Check sheet for the modelled part. Datum: model origin and axes. Units: mm. A direction names the side the tool comes from. Give positions to 0.01 mm unless a question says otherwise; leave off trailing zeros. Loops run counter-clockwise (first coordinate to the right, second up) from the corner with the lowest first, then second, coordinate; pieces in that order, holes last. Notation, with made-up numbers: (31, -18) -> (35, -18) arc R21 cw to (35, -1) -> close; hole circle Ø11 at (41, 33.5). An arc over 180 degrees is marked (long way). Write each question's results on one line, items separated by ' | '. Start each with the question number.
Item 1: Scan lines: line 1 along Z through (x, y) = (-4, 5); line 2 along Z through (x, y) = (12.5, 32.5); line 3 along X through (y, z) = (3.5, 3.75). Record each from-to range of solid material in increasing order.
Item 2: Cross-section at B-B on y = 37.5. Enter the section's corners in (x, z).
Item 3: Cross-section at A-A on x = 14. Enter the section's corners in (y, z).
Item 4: Cross-section at D-D on x = -2. Enter the section's corners in (y, z).
Item 5: Access from +Z, -Z, +X, -X, +Y, -Y to the whole of each face (thin tool, end or side, straight path). Record for faces 1 (the face through (0, 31, -8.25)), 2 (the face through (14, 22, -14.45)), 3 (the face through (-0.1, 12, 8.5)).
Item 6: Cross-section at C-C on z = -6.25. Enter the section's corners in (x, y).
Item 7: Mould release check, pull along Z, two halves, no side actions. Record for faces 4 (the face through (-14, 22, -14.45)), 5 (the face through (-7.65, 22.18, -10.76)), 6 (the face through (11.5, 22, -15)): pulls with the +Z half, pulls with the -Z half, needs draft (parallel to the pull), parting line crosses it, or undercut.
Item 8: Gauge pin test, flat ends, axial feed: pin 1 Ø12 at (x, z) = (-0.5, -12) entering from +Y; pin 2 Ø5 at (x, z) = (-2.5, -0.5) entering from +Y; pin 3 Ø3 at (x, y) = (6, 8.5) entering from -Z; pin 4 Ø1 at (y, z) = (14, 0.5) entering from -X (3 decimals). Record the tip position at first contact, or that the pin passes through.
from build123d import *

# Parameters (mm, degrees)
SKETCH1_W           = 39
SKETCH1_H           = 20.5
BOSS_EXTRUDE1_DEPTH = 2
SKETCH2_W           = 39
SKETCH2_H           = 20.5
SKETCH2_W_2         = 35
SKETCH2_H_2         = 16.5
BOSS_EXTRUDE2_DEPTH = 10
SKETCH3_W           = 39
SKETCH3_H           = 2
BOSS_EXTRUDE3_DEPTH = 48
FILLET1_R           = 10
FILLET2_R           = 1
BOSS_EXTRUDE4_DEPTH = 45


with BuildPart() as part:
    # Sketch1 → Boss-Extrude1 (new body)
    with BuildSketch(Plane(origin=(0, 0, 0), x_dir=(1, 0, 0), z_dir=(0, 1, 0))):
        Rectangle(SKETCH1_W, SKETCH1_H)
    extrude(amount=BOSS_EXTRUDE1_DEPTH)

    # Sketch2 → Boss-Extrude2 (add)
    with BuildSketch(Plane(origin=(0, 2, 0), x_dir=(1, 0, 0), z_dir=(0, 1, 0))):
        Rectangle(SKETCH2_W, SKETCH2_H)
        Rectangle(SKETCH2_W_2, SKETCH2_H_2, mode=Mode.SUBTRACT)
    extrude(amount=BOSS_EXTRUDE2_DEPTH)

    # Sketch3 → Boss-Extrude3 (add)
    with BuildSketch(Plane(origin=(0, 12, 0), x_dir=(1, 0, 0), z_dir=(0, 1, 0))):
        with Locations((0, 9.25)):
            Rectangle(SKETCH3_W, SKETCH3_H)
    extrude(amount=BOSS_EXTRUDE3_DEPTH)

    # Fillet1
    fillet1_edges = [part.edges().sort_by_distance(p)[0] for p in [
        (18.5, 12, -8.25),
        (-18.5, 12, -8.25),
    ]]
    fillet(fillet1_edges, radius=FILLET1_R)

    # Fillet2
    fillet2_edges = [part.edges().sort_by_distance(p)[0] for p in [
        (-17.5, 7, 8.25),
        (17.5, 7, 8.25),
        (17.5, 12, -8.25),
        (-17.5, 12, -8.25),
    ]]
    fillet(fillet2_edges, radius=FILLET2_R)

    # Sketch4 → Boss-Extrude4 (add)
    with BuildSketch(Plane.XZ):
        Polygon((-19.5, -10.25), (-19.5, -16.45), (-11.5, -16.45), (-11.5, -14.45), (-16.5, -14.45), (-16.5, -11.25), (-8.5, -11.25), (-6.767949192, -10.25), align=None)
    boss_extrude4 = extrude(amount=-BOSS_EXTRUDE4_DEPTH)

    # Mirror2: Boss-Extrude4 across plane
    add(boss_extrude4.mirror(Plane.ZY))


solid = part.part
Answer sheet:
1) line 1: z = -10.25 to -8.25, 8.25 to 10.25 | line 2: z = -16.45 to -14.45, -11.25 to -8.25 | line 3: x = -19.5 to -17.5, 17.5 to 19.5
2) outline: (-19.5, -16.45) -> (-11.5, -16.45) -> (-11.5, -14.45) -> (-16.5, -14.45) -> (-16.5, -11.25) -> (-8.5, -11.25) -> (-6.77, -10.25) -> (6.77, -10.25) -> (8.5, -11.25) -> (16.5, -11.25) -> (16.5, -14.45) -> (11.5, -14.45) -> (11.5, -16.45) -> (19.5, -16.45) -> (19.5, -8.25) -> (-19.5, -8.25) -> close
3) outline: (0, -16.45) -> (45, -16.45) -> (45, -14.45) -> (0, -14.45) -> close; (0, -11.25) -> (45, -11.25) -> (45, -10.25) -> (60, -10.25) -> (60, -8.25) -> (2, -8.25) -> (2, 8.25) -> (12, 8.25) -> (12, 10.25) -> (0, 10.25) -> close
4) outline: (0, -10.25) -> (60, -10.25) -> (60, -8.25) -> (2, -8.25) -> (2, 8.25) -> (12, 8.25) -> (12, 10.25) -> (0, 10.25) -> close
5) face 1: +Y | face 2: +Y, -Y | face 3: +Z, +X, -X, +Y
6) outline: (-19.5, 0) -> (19.5, 0) -> (19.5, 16) -> (17.5, 16) -> (17.5, 2) -> (-17.5, 2) -> (-17.5, 16) -> (-19.5, 16) -> close
7) face 4: undercut | face 5: pulls with the -Z half | face 6: needs draft
8) pin 1: stops at y = 60 | pin 2: stops at y = 2 | pin 3: stops at z = -10.67 | pin 4: passes through
